Here's how the part is built. I have some questions about the finished solid (model axes, mm). Face numbers are marked on the shaded views. A direction names the side the tool comes from. Round coordinates to 2 decimals unless told otherwise and drop trailing zeros. Loops run counter-clockwise (first coordinate to the right, second up) from the corner with the lowest first, then second, coordinate; pieces in that order, holes last. Notation, with made-up numbers: M -12.75,6.5 L 4.25,6.5 A33 cw 4.25,40.5 Z; hole C 30.5,-35.75 d1. An arc over 180 degrees is marked long. Write item = value, one per line. Start each with the question number.
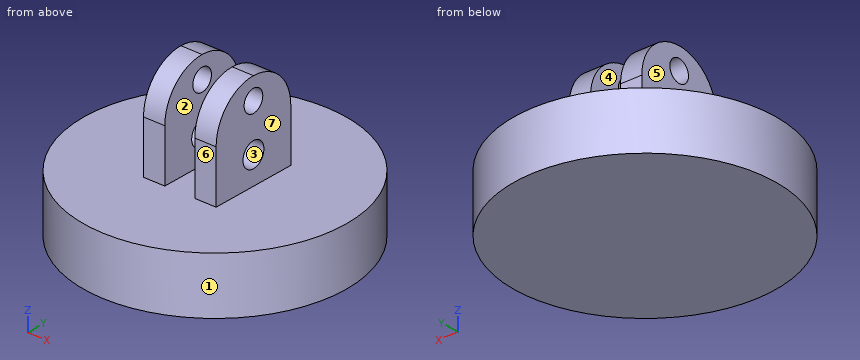
from build123d import *

# Parameters (mm, degrees)
F0_R     = 38.1
F1_DEPTH = 16.51
F2_W     = 6.20888776
F2_H     = 25.4
F2_W_2   = 6.2088776
F3_DEPTH = 27.94
F4_R     = 12.69999
F5_R     = 3.556
F5_R_2   = 3.175
F6_DEPTH = 49.319129452


# Not quite as in the source:
# - a fillet or chamfer is up to 0.001 mm smaller than in the source, because OpenCascade refuses the exact size


with BuildPart() as f1:
    # F0 (on Top) → F1 (new body)
    with BuildSketch(Plane.XY):
        Circle(F0_R)
    extrude(amount=F1_DEPTH)

    # F2 (on face) → F3 (join)
    with BuildSketch(Plane.XY.offset(16.51)):
        with Locations((-6.858192028, 0)):
            Rectangle(F2_W, F2_H)
        with Locations((8.113690652, 0)):
            Rectangle(F2_W_2, F2_H)
    extrude(amount=F3_DEPTH)

    # F4 (radius 12.7 in the source; OpenCascade refuses exactly that, so slightly less here)
    f4_edges = [f1.edges().sort_by_distance(p)[0] for p in [
        (-6.858192, 12.7, 44.45),
        (-6.858192, -12.7, 44.45),
        (8.113691, -12.7, 44.45),
        (8.113691, 12.7, 44.45),
    ]]
    fillet(f4_edges, radius=F4_R)

    # F5 (on face) → F6 (cut, through all)
    with BuildSketch(Plane.YZ.offset(11.218129452)):
        with Locations((0, 24.4883745909)):
            Circle(F5_R)
        with Locations((0, 38.0773745909)):
            Circle(F5_R_2)
    extrude(amount=-F6_DEPTH, mode=Mode.SUBTRACT)


solid = f1.part
Item 1: We'd pull the mould along X, two halves only. Please class the marked faces 1, 2, 3 and 4: released by +X, released by -X, zero draft, split by the parting line, or undercut.
Item 2: I want a section at B-B, the plane y = -11.5. List the corners of the cut face in (x, z) for me.
Item 3: Will these pins go through, and if not, where does the flat tip stop? pin 1 Ø1 at (y, z) = (-26.5, 19) entering from +X; pin 2 Ø3 at (y, z) = (-22.5, 10.5) entering from -X; pin 3 Ø20.5 at (y, z) = (1, 35) entering from -X; pin 4 Ø10 at (y, z) = (7, 24) entering from +X.
Item 4: Please list where these lines run through material, in increasing order: line 1 (Z direction, x = -8, y = 0); line 2 (X direction, y = 1.5, z = 17.5); line 3 (Z direction, x = 10.5, y = -18.5). Write a range as [from, to].
Item 5: I want a section at D-D, the plane x = 0. List the corners of the cut face in (y, z) for me.
Item 6: I want a section at C-C, the plane z = 26.5. List the corners of the cut face in (x, y) for me, then the cut area to 3 significant figures.
Item 7: I want a section at A-A, the plane z = 19.5. List the corners of the cut face in (x, y) for me.
Item 8: For the marked faces 5, 6 and 7, which set-ups out of +Z, -Z, +X, -X, +Y, -Y let a thin tool reach every point of the face, with its end or its side?
Worked out:
q1.face_1 = split by the parting line
q1.face_2 = undercut
q1.face_3 = zero draft
q1.face_4 = undercut
q2.outline = M -36.32,0 L 36.32,0 L 36.32,16.51 L 11.22,16.51 L 11.22,37.14 L 5.01,37.14 L 5.01,16.51 L -3.75,16.51 L -3.75,37.14 L -9.96,37.14 L -9.96,16.51 L -36.32,16.51 Z
q3.pin_1 = through
q3.pin_2 = -31.79
q3.pin_3 = -9.96
q3.pin_4 = 11.22
q4.line_1 = [0, 20.93], [28.04, 34.9], [41.25, 44.45]
q4.line_2 = [-9.96, -3.75], [5.01, 11.22]
q4.line_3 = [0, 16.51]
q5.outline = M -38.1,0 L 38.1,0 L 38.1,16.51 L -38.1,16.51 Z
q6.outline = M -9.96,-12.7 L -3.75,-12.7 L -3.75,-2.93 L -9.96,-2.93 Z; M -9.96,2.93 L -3.75,2.93 L -3.75,12.7 L -9.96,12.7 Z; M 5.01,-12.7 L 11.22,-12.7 L 11.22,-2.93 L 5.01,-2.93 Z; M 5.01,2.93 L 11.22,2.93 L 11.22,12.7 L 5.01,12.7 Z
q6.area = 243 mm2
q7.outline = M -9.96,-12.7 L -3.75,-12.7 L -3.75,12.7 L -9.96,12.7 Z; M 5.01,-12.7 L 11.22,-12.7 L 11.22,12.7 L 5.01,12.7 Z
q8.face_5 = +Z, -X, +Y, -Y
q8.face_6 = +Z, +X, -X, -Y
q8.face_7 = +Z, +X, +Y, -Y
